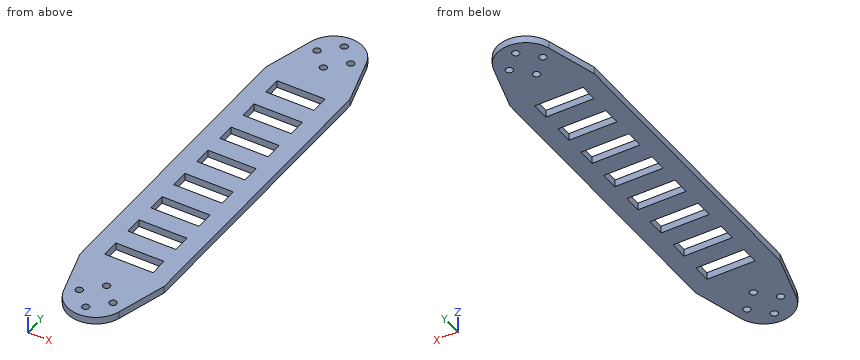
```python
from build123d import *

# Parameters (mm, degrees)
SKETCH1_R           = 1.5
SKETCH1_W           = 20
SKETCH1_H           = 7.5
BOSS_EXTRUDE4_DEPTH = 3


with BuildPart() as part:
    # Sketch1 → Boss-Extrude4 (new body)
    with BuildSketch(Plane.XY):
        with BuildLine():
            Line((-17.5, 142.5), (-17.5, 17.5))
            Line((-17.5, 17.5), (-11.535380853, -3.306809425))
            ThreePointArc((-11.535380853, -3.306809425), (0, -12), (11.535380853, -3.306809425))
            Line((11.535380853, -3.306809425), (17.5, 17.5))
            Line((17.5, 17.5), (17.5, 142.5))
            Line((17.5, 142.5), (11.535380853, 163.306809425))
            ThreePointArc((11.535380853, 163.306809425), (0, 172), (-11.535380853, 163.306809425))
            Line((-11.535380853, 163.306809425), (-17.5, 142.5))
        make_face()
        with Locations((-7, 0)):
            Circle(SKETCH1_R, mode=Mode.SUBTRACT)
        with Locations((0, 25.75)):
            Rectangle(SKETCH1_W, SKETCH1_H, mode=Mode.SUBTRACT)
        with Locations((0, -7)):
            Circle(SKETCH1_R, mode=Mode.SUBTRACT)
        with BuildLine():
            ThreePointArc((0, 8.5), (1.5, 7), (0, 5.5))
            ThreePointArc((0, 5.5), (-1.5, 7), (0, 8.5))
        make_face(mode=Mode.SUBTRACT)
        with Locations((7, 0)):
            Circle(SKETCH1_R, mode=Mode.SUBTRACT)
        with Locations((0, 41.25)):
            Rectangle(SKETCH1_W, SKETCH1_H, mode=Mode.SUBTRACT)
        with Locations((0, 56.75)):
            Rectangle(SKETCH1_W, SKETCH1_H, mode=Mode.SUBTRACT)
        with Locations((0, 72.25)):
            Rectangle(SKETCH1_W, SKETCH1_H, mode=Mode.SUBTRACT)
        with Locations((0, 87.75)):
            Rectangle(SKETCH1_W, SKETCH1_H, mode=Mode.SUBTRACT)
        with Locations((0, 103.25)):
            Rectangle(SKETCH1_W, SKETCH1_H, mode=Mode.SUBTRACT)
        with Locations((0, 118.75)):
            Rectangle(SKETCH1_W, SKETCH1_H, mode=Mode.SUBTRACT)
        with Locations((0, 134.25)):
            Rectangle(SKETCH1_W, SKETCH1_H, mode=Mode.SUBTRACT)
        with Locations((0, 167)):
            Circle(SKETCH1_R, mode=Mode.SUBTRACT)
        with BuildLine():
            ThreePointArc((0, 151.5), (-1.5, 153), (0, 154.5))
            ThreePointArc((0, 154.5), (1.5, 153), (0, 151.5))
        make_face(mode=Mode.SUBTRACT)
        with Locations((-7, 160)):
            Circle(SKETCH1_R, mode=Mode.SUBTRACT)
        with Locations((7, 160)):
            Circle(SKETCH1_R, mode=Mode.SUBTRACT)
    extrude(amount=BOSS_EXTRUDE4_DEPTH)


solid = part.part
```
For this review, take the finished solid that the model builds, in its own axes (mm). Coordinates: 2 decimals unless noted, no trailing zeros. Write each loop counter-clockwise with the first axis right and the second up, starting at its lowest first coordinate (ties: lowest second). Pieces come first, ordered by that corner, then holes.
(1) Add section B-B on y = 160. Give the boundary of the cut face in (x, z).
(2) For pin 1 Ø0.9 at (x, z) = (4, 1.5) entering from -Y; pin 2 Ø1.5 at (x, z) = (3, 1.5) entering from -Y; pin 3 Ø1.8 at (x, y) = (-7, 160) entering from +Z, all flat-tipped, find the tip position at first contact; note any pin that passes through.
(3) Add section A-A on y = 7. Give the boundary of the cut face in (x, z), then the cut area to 3 significant figures.
(4) Add section C-C on y = 26.5. Give the boundary of the cut face in (x, z), then the cut area to 3 significant figures.
(5) Wall thickness on probe 1 along X at (y, z) = (160, 0.8); probe 2 along X at (y, z) = (104, 1.05); probe 3 along X at (y, z) = (154, 2.8): over which ranges is each line inside the solid? List them lowest first.
(6) Add section D-D on x = 0. Count the separate pieces of the cut face and the enclosed holes in it, then the cut area to 3 significant figures.
Answer sheet:
1. outline: (-12.48, 0) - (-8.5, 0) - (-8.5, 3) - (-12.48, 3) - close; (-5.5, 0) - (5.5, 0) - (5.5, 3) - (-5.5, 3) - close; (8.5, 0) - (12.48, 0) - (12.48, 3) - (8.5, 3) - close
2. pin 1: stops at y = -11.46
2. pin 2: stops at y = -11.79
2. pin 3: passes through
3. outline: (-14.49, 0) - (-1.5, 0) - (-1.5, 3) - (-14.49, 3) - close; (1.5, 0) - (14.49, 0) - (14.49, 3) - (1.5, 3) - close
3. area: 77.9 mm2
4. outline: (-17.5, 0) - (-10, 0) - (-10, 3) - (-17.5, 3) - close; (10, 0) - (17.5, 0) - (17.5, 3) - (10, 3) - close
4. area: 45.0 mm2
5. probe 1: x = -12.48 to -8.5, -5.5 to 5.5, 8.5 to 12.48
5. probe 2: x = -17.5 to -10, 10 to 17.5
5. probe 3: x = -14.2 to -1.12, 1.12 to 14.2
6. separate pieces: 13
6. enclosed holes: 0
6. area: 336 mm2
